The model under review builds one solid part; all positions refer to its coordinate system, in mm. A direction names the side the tool comes from. Give positions to 0.01 mm unless a question says otherwise; leave off trailing zeros. Loops run counter-clockwise (first coordinate to the right, second up) from the corner with the lowest first, then second, coordinate; pieces in that order, holes last. Notation, with made-up numbers: (32, -20.75) -> (59, -20.75) arc R9 ccw to (59, -8.75) -> close; hole circle Ø6 at (67.5, -11). An arc over 180 degrees is marked (long way). Write each question's results on one line, items separated by ' | '. Start each with the question number.
Q1. Machinability: for faces 4 (the face through (-12.949, 4.93, 11.715)), 5 (the face through (9.37, 4.93, 10.45)), which of the approach directions +Z, -Z, +X, -X, +Y, -Y give a long, thin tool a straight path to every point of the face, cutting with its end or side? Answer none if there is none.
Q2. We need section C-C (y = 2). Write out the cut boundary in (x, z).
Q3. Insertion check: pin 1 Ø14.5 at (x, z) = (0, 0) entering from -Y (1 decimal); pin 2 Ø2 at (x, y) = (6.5, 7) entering from +Z; pin 3 Ø1.5 at (x, y) = (-9.5, 3.5) entering from +Z. Each pin has a flat end and moves straight along its axis. Give the tip position at first contact, or say it passes through.
Q4. Wall thickness on L1, parallel to X at y = 3.25, z = 0; L2, parallel to X at y = 4.5, z = 9.75; L3, parallel to Z at x = -0.5, y = 7.5: over which ranges is each line inside the solid? List them lowest first. Write a range as [from, to].
Q5. Mouldability with a two-part tool opening along Z and no side actions: class faces 1 (the face through (12.965, 4.93, 11.699)), 2 (the face through (12.949, 4.93, -16.215)), 3 (the face through (-9.33, 4.93, 10.37)) as released by +Z, released by -Z, zero draft, split by the parting line, or undercut.
Q6. We need section B-B (z = -10.25). Write out the cut boundary in (x, y), plus the area to 3 significant figures.
Q7. We need section D-D (x = 3). Write out the cut boundary in (y, z), plus the area to 3 significant figures.
Q8. We need section A-A (z = 0). Write out the cut boundary in (x, y), plus the area to 3 significant figures.
from build123d import *

# Parameters (mm, degrees)
BOSS_EXTRUDE1_DEPTH                             = 10
CSK_FOR_M2_FLAT_HEAD_MACHINE_SCREW1_D           = 2.4
CSK_FOR_M2_FLAT_HEAD_MACHINE_SCREW1_CSINK_D     = 4.4
CSK_FOR_M2_FLAT_HEAD_MACHINE_SCREW1_CSINK_ANGLE = 90


with BuildPart() as part:
    # Sketch1 → Boss-Extrude1 (new body)
    with BuildSketch(Plane(origin=(0, 0, 0), x_dir=(1, 0, 0), z_dir=(0, 1, 0))):
        with BuildLine():
            Line((12.25, -12), (12, -12))
            ThreePointArc((12, -12), (9.349555065, -10.408922304), (9.507567542, -7.321622732))
            ThreePointArc((9.507567542, -7.321622732), (0, 12), (-9.507567542, -7.321622732))
            ThreePointArc((-9.507567542, -7.321622732), (-9.349555065, -10.408922304), (-12, -12))
            Line((-12, -12), (-12.25, -12))
            ThreePointArc((-12.25, -12), (-12.957106781, -11.707106781), (-13.25, -11))
            Line((-13.25, -11), (-13.25, 15.5))
            ThreePointArc((-13.25, 15.5), (-12.957106781, 16.207106781), (-12.25, 16.5))
            Line((-12.25, 16.5), (12.25, 16.5))
            ThreePointArc((12.25, 16.5), (12.957106781, 16.207106781), (13.25, 15.5))
            Line((13.25, 15.5), (13.25, -11))
            ThreePointArc((13.25, -11), (12.957106781, -11.707106781), (12.25, -12))
        make_face()
    extrude(amount=BOSS_EXTRUDE1_DEPTH)

    # CSK for M2 Flat Head Machine Screw1 (through all)
    with Locations(Plane(origin=(-0.06607942, 5.031445439, -11.999818062), x_dir=(0.999984838462, 0, -0.005506618355), z_dir=(0.005506618355, 0, 0.999984838462))):
        with Locations((0, 0)):
            CounterSinkHole(CSK_FOR_M2_FLAT_HEAD_MACHINE_SCREW1_D / 2, CSK_FOR_M2_FLAT_HEAD_MACHINE_SCREW1_CSINK_D / 2, counter_sink_angle=CSK_FOR_M2_FLAT_HEAD_MACHINE_SCREW1_CSINK_ANGLE)


solid = part.part
Output:
1) face 4: +Z, -X, +Y, -Y | face 5: +Y, -Y
2) outline: (-13.25, -15.5) arc R1 ccw to (-12.25, -16.5) -> (12.25, -16.5) arc R1 ccw to (13.25, -15.5) -> (13.25, 11) arc R1 ccw to (12.25, 12) -> (12, 12) arc R3 ccw to (9.51, 7.32) arc R12 cw (long way) to (-9.51, 7.32) arc R3 ccw to (-12, 12) -> (-12.25, 12) arc R1 ccw to (-13.25, 11) -> close
3) pin 1: through | pin 2: z = -9.37 | pin 3: z = 11.44
4) L1: [-13.25, -12], [12, 13.25] | L2: [-13.25, -9.09], [9.09, 13.25] | L3: [-16.5, -11.99]
5) face 1: released by +Z | face 2: released by -Z | face 3: undercut
6) outline: (-13.25, 0) -> (-6.24, 0) -> (-6.24, 10) -> (-13.25, 10) -> close; (6.24, 0) -> (13.25, 0) -> (13.25, 10) -> (6.24, 10) -> close | area: 140 mm2
7) outline: (0, -16.5) -> (10, -16.5) -> (10, -11.62) -> (0, -11.62) -> close | area: 48.8 mm2
8) outline: (-13.25, 0) -> (-12, 0) -> (-12, 10) -> (-13.25, 10) -> close; (12, 0) -> (13.25, 0) -> (13.25, 10) -> (12, 10) -> close | area: 25.0 mm2
